Read the model definition and answer for the solid it produces. Units are mm, in the model's axes. Coordinates: 2 decimals unless noted, no trailing zeros. Order: outer loops, then holes, each group sorted by start corner. A loop starts at its lowest first (then second) coordinate and runs counter-clockwise, first axis right, second up.
```python
from build123d import *

# Parameters (mm, degrees)
BOSS_EXTRUDE1_DEPTH = 0.3
SKETCH7_R           = 1.905
CUT_EXTRUDE3_DEPTH  = 68.232035618
CUT_EXTRUDE4_DEPTH  = 68.232035618


with BuildPart() as part:
    # Sketch5 → Boss-Extrude1 (new body)
    with BuildSketch(Plane.XY):
        with BuildLine():
            Line((-2.028916314, 32.899205852), (-3.033121883, 49.182561418))
            ThreePointArc((-3.033121883, 49.182561418), (-28.963706092, 39.865121415), (-45.838109317, 18.082917637))
            Line((-45.838109317, 18.082917637), (-30.662034486, 12.096027791))
            Line((-30.662034486, 12.096027791), (-18.848088785, 7.435482008))
            Line((-18.848088785, 7.435482008), (-7.679064705, 3.029354759))
            ThreePointArc((-7.679064705, 3.029354759), (-4.852167258, 6.678435289), (-0.508126089, 8.239346629))
            Line((-0.508126089, 8.239346629), (-1.24718387, 20.223287961))
            Line((-1.24718387, 20.223287961), (-2.028916314, 32.899205852))
        make_face()
    extrude(amount=BOSS_EXTRUDE1_DEPTH)

    # Sketch7 → Cut-Extrude3 (cut, through all)
    with BuildSketch(Plane(origin=(0, 0, 0), x_dir=(-1, 0, 0), z_dir=(0, 0, -1))):
        with Locations((26.831076285, 36.924921792)):
            Circle(SKETCH7_R)
        with Locations((19.375810402, 26.663628618)):
            Circle(SKETCH7_R)
    extrude(amount=-CUT_EXTRUDE3_DEPTH, mode=Mode.SUBTRACT)

    # Sketch8 → Cut-Extrude4 (cut, through all)
    with BuildSketch(Plane(origin=(0, 0, 0), x_dir=(-1, 0, 0), z_dir=(0, 0, -1))):
        with BuildLine():
            Line((1.290332778, 20.922954474), (1.933991563, 31.359985686))
            ThreePointArc((1.933991563, 31.359985686), (5.427783746, 25.906158112), (1.290332778, 20.922954474))
        make_face()
        with BuildLine():
            Line((29.233104835, 11.532321793), (19.432314115, 7.665956142))
            ThreePointArc((19.432314115, 7.665956142), (22.882252084, 13.27588106), (29.233104835, 11.532321793))
        make_face()
    extrude(amount=-CUT_EXTRUDE4_DEPTH, mode=Mode.SUBTRACT)


solid = part.part
```
1) Flat-ended cylindrical pins translate along their axes: pin 1 Ø1 at (x, y) = (-23, 40.5) entering from -Z; pin 2 Ø10 at (x, y) = (-34.5, 42) entering from -Z. Find the tip coordinate at first contact, or state that the pin passes through.
A:
pin 1: stops at z = 0
pin 2: passes through
2) A cutting plane is placed at C-C, the plane x = -9.5. Determine the outline of the cut face in (y, z).
A:
outline: (3.75, 0) - (48.35, 0) - (48.35, 0.3) - (3.75, 0.3) - close
3) Determine the mould class of faces 1 (the cylindrical face through (-21.19, 27.24, 0.15)), 2 (the flat face through (-13, 26, 0)) for opening direction X: pulls with the +X half, pulls with the -X half, needs draft (parallel to the pull), parting line crosses it, or undercut.
A:
face 1: undercut
face 2: needs draft
4) Straight lines are drawn through the part: line 1 (Y direction, x = -4.5, z = 0.15); line 2 (Y direction, x = -18.5, z = 0.1); line 3 (X direction, y = 43, z = 0.1) (3 decimals). For each, find the intervals that lie inside material, in ascending order.
A:
line 1: y = 6.92 to 23.18, 29.31 to 49.07
line 2: y = 7.3 to 24.97, 28.36 to 45.67
line 3: x = -24.065 to -2.652
5) A cutting plane is placed at D-D, the plane y = 30.5. Determine the outline of the cut face in (x, z).
A:
outline: (-38.7, 0) - (-3.41, 0) - (-3.41, 0.3) - (-38.7, 0.3) - close
6) A cutting plane is placed at A-A, the plane y = 37.5. Determine the outline of the cut face in (x, z).
A:
outline: (-31.97, 0) - (-28.65, 0) - (-28.65, 0.3) - (-31.97, 0.3) - close; (-25.01, 0) - (-2.31, 0) - (-2.31, 0.3) - (-25.01, 0.3) - close
7) A cutting plane is placed at B-B, the plane z = 0.1. Determine the outline of the cut face in (x, y) (3 decimals).
A:
outline: (-45.838, 18.083) - (-29.233, 11.532) arc R5.487 cw to (-19.432, 7.666) - (-7.679, 3.029) arc R8.255 cw to (-0.508, 8.239) - (-1.29, 20.923) arc R5.487 cw to (-1.934, 31.36) - (-3.033, 49.183) arc R49.276 ccw to start; hole circle Ø3.81 at (-26.831, 36.925); hole circle Ø3.81 at (-19.376, 26.664)
